Source: CAD feature listing. Evaluate the final solid. Frame: model axes, mm. Give positions to 0.01 mm unless a question says otherwise; leave off trailing zeros. Order: outer loops, then holes, each group sorted by start corner. A loop starts at its lowest first (then second) coordinate and runs counter-clockwise, first axis right, second up. Notation, with made-up numbers: (67.25, -10.5) - (104.25, -10.5) arc R6 cw to (104.25, -0.5) - close; hole circle Ø2 at (45, 85). An arc over 180 degrees is marked (long way). Write each question's results on one line, items separated by ' | '. Start each with the question number.
Item 1: Section A-A on y = 97.5. Output: boundary loops of the cut face in (x, z), and give its area (3 significant figures).
Item 2: Section C-C on z = 1.9. State how many separate pieces and enclosed holes the cut face has, and give its area (3 significant figures).
Item 3: Contact query for a flat-ended pin moving along its axis: pin 1 Ø2.5 at (x, y) = (-65.44, 74.06) entering from +Z. Output: stop coordinate, or through.
Item 4: Line query: line 1 along X through (y, z) = (68, 2); line 2 along Y through (x, z) = (-86.5, 2.05); line 3 along Y through (x, z) = (-20, 1.4). Output: solid intervals per line, ascending.
Item 5: Section B-B on x = -41. Output: boundary loops of the cut face in (y, z).
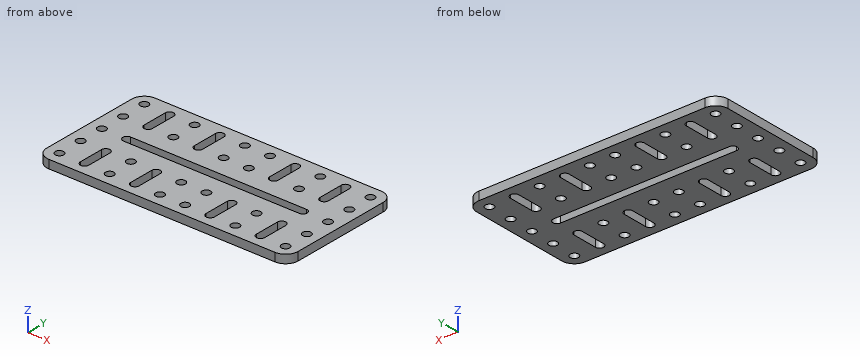
```python
from build123d import *

# Parameters (mm, degrees)
MODEL_R                 = 1.5
SALIENTE_EXTRUIR1_DEPTH = 3


with BuildPart() as part:
    # Model → Saliente-Extruir1 (new body)
    with BuildSketch(Plane.XY):
        with BuildLine():
            Line((-105.943383637, 101.056539338), (-105.943383637, 65.056539338))
            ThreePointArc((-105.943383637, 65.056539338), (-104.625364152, 61.874558823), (-101.443383637, 60.556539338))
            Line((-101.443383637, 60.556539338), (-20.443383637, 60.556539338))
            ThreePointArc((-20.443383637, 60.556539338), (-17.261403122, 61.874558823), (-15.943383637, 65.056539338))
            Line((-15.943383637, 65.056539338), (-15.943383637, 101.056539338))
            ThreePointArc((-15.943383637, 101.056539338), (-17.261403122, 104.238519853), (-20.443383637, 105.556539338))
            Line((-20.443383637, 105.556539338), (-101.443383637, 105.556539338))
            ThreePointArc((-101.443383637, 105.556539338), (-104.625364152, 104.238519853), (-105.943383637, 101.056539338))
        make_face()
        with Locations((-101.443383637, 101.056539338)):
            Circle(MODEL_R, mode=Mode.SUBTRACT)
        with Locations((-83.443383637, 101.056539338)):
            Circle(MODEL_R, mode=Mode.SUBTRACT)
        with Locations((-65.443383637, 101.056539338)):
            Circle(MODEL_R, mode=Mode.SUBTRACT)
        with Locations((-56.443383637, 101.056539338)):
            Circle(MODEL_R, mode=Mode.SUBTRACT)
        with Locations((-38.443383637, 101.056539338)):
            Circle(MODEL_R, mode=Mode.SUBTRACT)
        with Locations((-101.443383637, 92.056539338)):
            Circle(MODEL_R, mode=Mode.SUBTRACT)
        with Locations((-83.443383637, 92.056539338)):
            Circle(MODEL_R, mode=Mode.SUBTRACT)
        with Locations((-65.443383637, 92.056539338)):
            Circle(MODEL_R, mode=Mode.SUBTRACT)
        with Locations((-56.443383637, 92.056539338)):
            Circle(MODEL_R, mode=Mode.SUBTRACT)
        with Locations((-38.443383637, 92.056539338)):
            Circle(MODEL_R, mode=Mode.SUBTRACT)
        with Locations((-101.443383637, 83.056539338)):
            Circle(MODEL_R, mode=Mode.SUBTRACT)
        with Locations((-101.443383637, 65.056539338)):
            Circle(MODEL_R, mode=Mode.SUBTRACT)
        with Locations((-83.443383637, 65.056539338)):
            Circle(MODEL_R, mode=Mode.SUBTRACT)
        with Locations((-65.443383637, 65.056539338)):
            Circle(MODEL_R, mode=Mode.SUBTRACT)
        with Locations((-56.443383637, 65.056539338)):
            Circle(MODEL_R, mode=Mode.SUBTRACT)
        with Locations((-38.443383637, 65.056539338)):
            Circle(MODEL_R, mode=Mode.SUBTRACT)
        with Locations((-20.443383637, 101.056539338)):
            Circle(MODEL_R, mode=Mode.SUBTRACT)
        with Locations((-20.443383637, 92.056539338)):
            Circle(MODEL_R, mode=Mode.SUBTRACT)
        with Locations((-20.443383637, 83.056539338)):
            Circle(MODEL_R, mode=Mode.SUBTRACT)
        with Locations((-20.443383637, 65.056539338)):
            Circle(MODEL_R, mode=Mode.SUBTRACT)
        with Locations((-101.443383637, 74.056539338)):
            Circle(MODEL_R, mode=Mode.SUBTRACT)
        with Locations((-83.443383637, 74.056539338)):
            Circle(MODEL_R, mode=Mode.SUBTRACT)
        with Locations((-65.443383637, 74.056539338)):
            Circle(MODEL_R, mode=Mode.SUBTRACT)
        with Locations((-56.443383637, 74.056539338)):
            Circle(MODEL_R, mode=Mode.SUBTRACT)
        with Locations((-38.443383637, 74.056539338)):
            Circle(MODEL_R, mode=Mode.SUBTRACT)
        with Locations((-20.443383637, 74.056539338)):
            Circle(MODEL_R, mode=Mode.SUBTRACT)
        with BuildLine():
            Line((-92.443383637, 84.556539338), (-29.443383637, 84.556539338))
            ThreePointArc((-29.443383637, 84.556539338), (-27.943383637, 83.056539338), (-29.443383637, 81.556539338))
            Line((-29.443383637, 81.556539338), (-92.443383637, 81.556539338))
            ThreePointArc((-92.443383637, 81.556539338), (-93.943383637, 83.056539338), (-92.443383637, 84.556539338))
        make_face(mode=Mode.SUBTRACT)
        with BuildLine():
            Line((-93.943383637, 74.056539338), (-93.943383637, 65.056539338))
            ThreePointArc((-93.943383637, 65.056539338), (-92.443383637, 63.556539338), (-90.943383637, 65.056539338))
            Line((-90.943383637, 65.056539338), (-90.943383637, 74.056539338))
            ThreePointArc((-90.943383637, 74.056539338), (-92.443383637, 75.556539338), (-93.943383637, 74.056539338))
        make_face(mode=Mode.SUBTRACT)
        with BuildLine():
            Line((-75.943383637, 74.056539338), (-75.943383637, 65.056539338))
            ThreePointArc((-75.943383637, 65.056539338), (-74.443383637, 63.556539338), (-72.943383637, 65.056539338))
            Line((-72.943383637, 65.056539338), (-72.943383637, 74.056539338))
            ThreePointArc((-72.943383637, 74.056539338), (-74.443383637, 75.556539338), (-75.943383637, 74.056539338))
        make_face(mode=Mode.SUBTRACT)
        with BuildLine():
            Line((-48.943383637, 74.056539338), (-48.943383637, 65.056539338))
            ThreePointArc((-48.943383637, 65.056539338), (-47.443383637, 63.556539338), (-45.943383637, 65.056539338))
            Line((-45.943383637, 65.056539338), (-45.943383637, 74.056539338))
            ThreePointArc((-45.943383637, 74.056539338), (-47.443383637, 75.556539338), (-48.943383637, 74.056539338))
        make_face(mode=Mode.SUBTRACT)
        with BuildLine():
            Line((-30.943383637, 74.056539338), (-30.943383637, 65.056539338))
            ThreePointArc((-30.943383637, 65.056539338), (-29.443383637, 63.556539338), (-27.943383637, 65.056539338))
            Line((-27.943383637, 65.056539338), (-27.943383637, 74.056539338))
            ThreePointArc((-27.943383637, 74.056539338), (-29.443383637, 75.556539338), (-30.943383637, 74.056539338))
        make_face(mode=Mode.SUBTRACT)
        with BuildLine():
            Line((-93.943383637, 101.056539338), (-93.943383637, 92.056539338))
            ThreePointArc((-93.943383637, 92.056539338), (-92.443383637, 90.556539338), (-90.943383637, 92.056539338))
            Line((-90.943383637, 92.056539338), (-90.943383637, 101.056539338))
            ThreePointArc((-90.943383637, 101.056539338), (-92.443383637, 102.556539338), (-93.943383637, 101.056539338))
        make_face(mode=Mode.SUBTRACT)
        with BuildLine():
            Line((-75.943383637, 101.056539338), (-75.943383637, 92.056539338))
            ThreePointArc((-75.943383637, 92.056539338), (-74.443383637, 90.556539338), (-72.943383637, 92.056539338))
            Line((-72.943383637, 92.056539338), (-72.943383637, 101.056539338))
            ThreePointArc((-72.943383637, 101.056539338), (-74.443383637, 102.556539338), (-75.943383637, 101.056539338))
        make_face(mode=Mode.SUBTRACT)
        with BuildLine():
            Line((-48.943383637, 101.056539338), (-48.943383637, 92.056539338))
            ThreePointArc((-48.943383637, 92.056539338), (-47.443383637, 90.556539338), (-45.943383637, 92.056539338))
            Line((-45.943383637, 92.056539338), (-45.943383637, 101.056539338))
            ThreePointArc((-45.943383637, 101.056539338), (-47.443383637, 102.556539338), (-48.943383637, 101.056539338))
        make_face(mode=Mode.SUBTRACT)
        with BuildLine():
            Line((-30.943383637, 101.056539338), (-30.943383637, 92.056539338))
            ThreePointArc((-30.943383637, 92.056539338), (-29.443383637, 90.556539338), (-27.943383637, 92.056539338))
            Line((-27.943383637, 92.056539338), (-27.943383637, 101.056539338))
            ThreePointArc((-27.943383637, 101.056539338), (-29.443383637, 102.556539338), (-30.943383637, 101.056539338))
        make_face(mode=Mode.SUBTRACT)
    extrude(amount=SALIENTE_EXTRUIR1_DEPTH)


solid = part.part
```
Evaluation:
1) outline: (-105.94, 0) - (-93.94, 0) - (-93.94, 3) - (-105.94, 3) - close; (-90.94, 0) - (-75.94, 0) - (-75.94, 3) - (-90.94, 3) - close; (-72.94, 0) - (-48.94, 0) - (-48.94, 3) - (-72.94, 3) - close; (-45.94, 0) - (-30.94, 0) - (-30.94, 3) - (-45.94, 3) - close; (-27.94, 0) - (-15.94, 0) - (-15.94, 3) - (-27.94, 3) - close | area: 234 mm^2
2) separate pieces: 1 | enclosed holes: 35 | area: 3,380 mm^2
3) pin 1: passes through
4) line 1: x = -105.94 to -93.94, -90.94 to -75.94, -72.94 to -48.94, -45.94 to -30.94, -27.94 to -15.94 | line 2: y = 60.56 to 81.56, 84.56 to 105.56 | line 3: y = 60.58 to 63.62, 66.49 to 72.62, 75.49 to 81.62, 84.49 to 90.62, 93.49 to 99.62, 102.49 to 105.53
5) outline: (60.56, 0) - (81.56, 0) - (81.56, 3) - (60.56, 3) - close; (84.56, 0) - (105.56, 0) - (105.56, 3) - (84.56, 3) - close
